The model under review builds one solid part; all positions refer to its coordinate system, in mm. A direction names the side the tool comes from. Give positions to 0.01 mm unless a question says otherwise; leave off trailing zeros. Order: outer loops, then holes, each group sorted by start corner. A loop starts at its lowest first (then second) coordinate and runs counter-clockwise, first axis right, second up. Notation, with made-up numbers: (-25, 18.25) - (12, 18.25) arc R16 cw to (12, 24.25) - close; hole circle Ø4 at (-34, 81). An arc over 180 degrees is marked (long way). Put each result on its own line as item: value.
Autodesk Inventor part; units mm, degrees
ref_plane "YZ Plane" through (0, 0, 0) normal (1, 0, 0) x (0, 1, 0)
ref_plane "XZ Plane" through (0, 0, 0) normal (0, 1, 0) x (-1, 0, 0)
ref_plane "XY Plane" through (0, 0, 0) normal (0, 0, 1) x (1, 0, 0)
sketch "Sketch1" plane through (0, 0, 0) normal (1, 0, 0) x (0, 1, 0)
  line L0 (0, 0) -> (-36.5, 0)
  line L1 (-40, -3.5) -> (-40, -14.5)
  line L2 (-36.5, -18) -> (0, -18)
  line L3 (0, -18) -> (0, 0)
  line L4 (-13.5, -5.5) -> (-33.5, -5.5)
  line L5 (-37, -9) -> (-37, -9)
  line L6 (-33.5, -12.5) -> (-13.5, -12.5)
  line L7 (-10, -9) -> (-10, -9)
  arc A0 (-37, -9) -> (-33.5, -12.5) centre (-33.5, -9) ccw
  arc A1 (-33.5, -5.5) -> (-37, -9) centre (-33.5, -9) ccw
  arc A2 (-10, -9) -> (-13.5, -5.5) centre (-13.5, -9) ccw
  arc A3 (-13.5, -12.5) -> (-10, -9) centre (-13.5, -9) ccw
  arc A4 (-36.5, 0) -> (-40, -3.5) centre (-36.5, -3.5) ccw
  arc A5 (-40, -14.5) -> (-36.5, -18) centre (-36.5, -14.5) ccw
  point P0 (-40, -18)
  point P1 (-10, -5.5)
  point P2 (-37, -12.5)
  point P3 (-10, -12.5)
  dimension "d0" = 40
  dimension "d1" = 18
  dimension "d2" = 27
  dimension "d3" = 7
  dimension "d4" = 5.5
  dimension "d5" = 10
  dimension "d6" = 3.5
extrude "Extrusion1" add sketch "Sketch1" along normal blind 3
sketch "Sketch2" plane through (3, 0, 0) normal (1, 0, 0) x (0, 0, -1)
  line L0 (18, 0) -> (0, 0)
  line L1 (0, 0) -> (0, -36.5)
  line L2 (18, -36.5) -> (18, 0)
  point P0 (3, -2)
  point P1 (15, -2)
  dimension "d9" = 2
  dimension "d10" = 2
  dimension "d11" = 3
  dimension "d12" = 3
hole "Hole1" at (3, -2, -3) at (3, -2, -15) direction (-1, 0, 0) diameter 2.4 depth 8.8 tip angle 118
chamfer "Chamfer1" distance 0.3 angle 45 26 edges at (0, 0, -9) (3, 0, -9) (1.5, 0, 0) (3, -18.25, 0) (3, -38.9749, -1.0251) (3, -40, -9) (3, -38.9749, -16.9749) (3, -18.25, -18) (0, -18.25, 0) (0, -38.9749, -1.0251) (0, -40, -9) (0, -38.9749, -16.9749) (0, -18.25, -18) (3, -2, -13.8) (3, -2, -1.8) (3, -10, -9) (3, -23.5, -12.5) (3, -37, -9) (3, -23.5, -5.5) (0, -23.5, -12.5) (0, -10, -9) (0, -23.5, -5.5) (0, -37, -9) (1.5, 0, -18) (0, -2, -13.8) (0, -2, -1.8)
properties part number "Ramka2" material "Steel(1)"
(1) The part is to be moulded in two halves that separate along Z. For faces 1 (the flat face through (3, -20, -5)), 2 (the cylindrical face through (1.48, -3.01, -15.65)), 3 (the conical face through (0.119, -38.872, -16.821)), say which applies: pulls with the +Z half, pulls with the -Z half, needs draft (parallel to the pull), parting line crosses it, or undercut.
The answers:
face 1: needs draft
face 2: undercut
face 3: pulls with the -Z half
(2) Take a section at B-B, the plane z = -9. Write out the cut boundary in (x, y), then the cut area to 3 significant figures.
The answers:
outline: (0, -39.7) - (0.3, -40) - (2.7, -40) - (3, -39.7) - (3, -37.3) - (2.7, -37) - (0.3, -37) - (0, -37.3) - close; (0, -9.7) - (0.3, -10) - (2.7, -10) - (3, -9.7) - (3, -0.3) - (2.7, 0) - (0.3, 0) - (0, -0.3) - close
area: 38.6 mm^2
(3) Wall thickness on L1, parallel to Z at x = 1, y = -2; L2, parallel to Z at x = 1.3, y = -33; L3, parallel to Y at x = 0.6, z = -10.5: over which ranges is each line inside the solid? List them lowest first.
The answers:
L1: -18 to -16.2, -13.8 to -4.2, -1.8 to 0
L2: -18 to -12.5, -5.5 to 0
L3: -40 to -36.66, -10.34 to 0
(4) Take a section at C-C, the plane y = -2. Write out the cut boundary in (x, z).
The answers:
outline: (0, -17.7) - (0.3, -18) - (2.7, -18) - (3, -17.7) - (3, -16.5) - (2.7, -16.2) - (0.3, -16.2) - (0, -16.5) - close; (0, -13.5) - (0.3, -13.8) - (2.7, -13.8) - (3, -13.5) - (3, -4.5) - (2.7, -4.2) - (0.3, -4.2) - (0, -4.5) - close; (0, -1.5) - (0.3, -1.8) - (2.7, -1.8) - (3, -1.5) - (3, -0.3) - (2.7, 0) - (0.3, 0) - (0, -0.3) - close
(5) For faces 4 (the flat face through (1, -24, -12.5)), 5 (the conical face through (2.82, -9.88, -9.08)), 6 (the conical face through (0.18, -37.12, -9.08)), 7 (the conical face through (2.881, -38.872, -1.179)), list the 3-axis set-ups (+Z, -Z, +X, -X, +Y, -Y) from which the entire face can be reached by the end or side of a thin tool; tool diameter is ignored.
The answers:
face 4: +X, -X
face 5: +X
face 6: -X
face 7: +Z, +X, -Y
(6) Take a section at D-D, the plane x = 2.2. Write out the cut boundary in (y, z), then the cut area to 3 significant figures.
The answers:
outline: (-40, -14.5) arc R3.5 ccw to (-36.5, -18) - (-0.3, -18) - (0, -17.7) - (0, -0.3) - (-0.3, 0) - (-36.5, 0) arc R3.5 ccw to (-40, -3.5) - close; hole (-33.5, -12.5) - (-13.5, -12.5) arc R3.5 ccw to (-13.5, -5.5) - (-33.5, -5.5) arc R3.5 ccw to start; hole circle Ø2.4 at (-2, -15); hole circle Ø2.4 at (-2, -3)
area: 527 mm^2
(7) Take a section at A-A, the plane y = -20.5. Write out the cut boundary in (x, z).
The answers:
outline: (0, -17.7) - (0.3, -18) - (2.7, -18) - (3, -17.7) - (3, -12.8) - (2.7, -12.5) - (0.3, -12.5) - (0, -12.8) - close; (0, -5.2) - (0.3, -5.5) - (2.7, -5.5) - (3, -5.2) - (3, -0.3) - (2.7, 0) - (0.3, 0) - (0, -0.3) - close
